from build123d import *

# Parameters (mm, degrees)
BOSS_EXTRUDE1_DEPTH      = 70
BOSS_EXTRUDE1_DEPTH_BACK = 70
SKETCH1_W                = 20
SKETCH1_H                = 10
SKETCH3_W                = 20
SKETCH3_H                = 5
BOSS_EXTRUDE2_DEPTH      = 20
FILLET1_R                = 10
SKETCH4_R                = 2.75
CUT_EXTRUDE1_DEPTH       = 91.863909227
FILLET1_OF_MIRROR1_R     = 10
CHAMFER1_SIZE            = 8.660254038
CHAMFER1_SIZE_2          = 5


# Some blends are built 0.0001 mm under size
with BuildPart() as part:
    # Sketch1 → Boss-Extrude1 (new, two sides: drawn at the far end of the back side and taken through both)
    with BuildSketch(Plane.XY.offset(-BOSS_EXTRUDE1_DEPTH_BACK)):
        Rectangle(SKETCH1_W, SKETCH1_H)
    extrude(amount=BOSS_EXTRUDE1_DEPTH + BOSS_EXTRUDE1_DEPTH_BACK)

    # Sketch3 → Boss-Extrude2 (add)
    with BuildSketch(Plane(origin=(0, 0, -70), x_dir=(-1, 0, 0), z_dir=(0, 0, -1))):
        Rectangle(SKETCH3_W, SKETCH3_H)
    boss_extrude2 = extrude(amount=BOSS_EXTRUDE2_DEPTH)

    # Fillet1
    fillet1_edges = [part.edges().sort_by_distance(p)[0] for p in [
        (-10, 0, -90),
        (10, 0, -90),
    ]]
    fillet(fillet1_edges, radius=FILLET1_R - 0.0001)  # a hair under: the kernel refuses the full size

    # Sketch4 → Cut-Extrude1 (cut, through all)
    with BuildSketch(Plane(origin=(0, 2.5, 0), x_dir=(1, 0, 0), z_dir=(0, 1, 0))):
        with Locations(Location((0, 80, 0), (0, 0, 270))):
            Circle(SKETCH4_R)
    cut_extrude1 = extrude(amount=-CUT_EXTRUDE1_DEPTH, mode=Mode.SUBTRACT)

    # Mirror1: Boss-Extrude2, Cut-Extrude1 across plane
    add(boss_extrude2.mirror(Plane.XY))
    add(cut_extrude1.mirror(Plane.XY), mode=Mode.SUBTRACT)

    # Fillet1 of Mirror1
    fillet1_of_mirror1_edges = [part.edges().sort_by_distance(p)[0] for p in [
        (-10, 0, 90),
        (10, 0, 90),
    ]]
    fillet(fillet1_of_mirror1_edges, radius=FILLET1_OF_MIRROR1_R - 0.0001)  # a hair under: the kernel refuses the full size

    # Chamfer1
    # the kernel refuses this chamfer: 8.660254038, 5 mm, written as the material it takes off along each edge
    with BuildSketch(Plane(origin=(32.404819853, 5, -70), x_dir=(0, 0.019326765612700594, 0.999813220622208), z_dir=(-1, 0, 0))) as chamfer1_piece_1_section:
        Polygon((CHAMFER1_SIZE * 0.999813220604, -CHAMFER1_SIZE * 0.0193267656124), (-CHAMFER1_SIZE_2 * 0.0193267656127, -CHAMFER1_SIZE_2 * 0.999813220622), (0, 0), align=None)
    chamfer1_piece_1 = extrude(amount=64.809639706, mode=Mode.PRIVATE)
    chamfer1_piece_1 = split(chamfer1_piece_1, bisect_by=Plane(origin=(0, 2.5, -66.539331058), z_dir=(0, 1, 0)), keep=Keep.TOP, mode=Mode.PRIVATE)
    add(chamfer1_piece_1, mode=Mode.SUBTRACT)
    with BuildSketch(Plane(origin=(-32.404819853, -5, -70), x_dir=(0, -0.019326765612700594, 0.999813220622208), z_dir=(1, 0, 0))) as chamfer1_piece_2_section:
        Polygon((CHAMFER1_SIZE * 0.999813220604, -CHAMFER1_SIZE * 0.0193267656124), (-CHAMFER1_SIZE_2 * 0.0193267656127, -CHAMFER1_SIZE_2 * 0.999813220622), (0, 0), align=None)
    chamfer1_piece_2 = extrude(amount=64.809639706, mode=Mode.PRIVATE)
    chamfer1_piece_2 = split(chamfer1_piece_2, bisect_by=Plane(origin=(0, -2.5, -66.539331058), z_dir=(0, -1, 0)), keep=Keep.TOP, mode=Mode.PRIVATE)
    add(chamfer1_piece_2, mode=Mode.SUBTRACT)
    with BuildSketch(Plane(origin=(-32.404819853, -5, 70), x_dir=(0, 0.9983227437537926, 0.05789386240267045), z_dir=(1, 0, 0))) as chamfer1_piece_3_section:
        Polygon((CHAMFER1_SIZE_2 * 0.998322743754, -CHAMFER1_SIZE_2 * 0.0578938624027), (-CHAMFER1_SIZE * 0.0578938624016, -CHAMFER1_SIZE * 0.998322743736), (0, 0), align=None)
    chamfer1_piece_3 = extrude(amount=64.809639706, mode=Mode.PRIVATE)
    chamfer1_piece_3 = split(chamfer1_piece_3, bisect_by=Plane(origin=(0, -2.5, 66.539331058), z_dir=(0, -1, 0)), keep=Keep.TOP, mode=Mode.PRIVATE)
    add(chamfer1_piece_3, mode=Mode.SUBTRACT)
    with BuildSketch(Plane(origin=(32.404819853, 5, 70), x_dir=(0, -0.9983227437537926, 0.05789386240267045), z_dir=(-1, 0, 0))) as chamfer1_piece_4_section:
        Polygon((CHAMFER1_SIZE_2 * 0.998322743754, -CHAMFER1_SIZE_2 * 0.0578938624027), (-CHAMFER1_SIZE * 0.0578938624016, -CHAMFER1_SIZE * 0.998322743736), (0, 0), align=None)
    chamfer1_piece_4 = extrude(amount=64.809639706, mode=Mode.PRIVATE)
    chamfer1_piece_4 = split(chamfer1_piece_4, bisect_by=Plane(origin=(0, 2.5, 66.539331058), z_dir=(0, 1, 0)), keep=Keep.TOP, mode=Mode.PRIVATE)
    add(chamfer1_piece_4, mode=Mode.SUBTRACT)


solid = part.part
Check sheet for the modelled part. Datum: model origin and axes. Units: mm. A direction names the side the tool comes from. Coordinates: 2 decimals unless noted, no trailing zeros. Write each loop counter-clockwise with the first axis right and the second up, starting at its lowest first coordinate (ties: lowest second). Pieces come first, ordered by that corner, then holes.
Item 1: Access from +Z, -Z, +X, -X, +Y, -Y to the whole of each face (thin tool, end or side, straight path). Record for faces 1 (the face through (0, 2.5, -75)), 2 (the face through (0, -2.5, -75)), 3 (the face through (0, -2.5, 75)), 4 (the face through (0, 2.5, 75)).
Numbers:
face 1: -Z, +X, -X, +Y
face 2: -Z, +X, -X, -Y
face 3: +Z, +X, -X, -Y
face 4: +Z, +X, -X, +Y
Item 2: Scan lines: probe 1 along X at (y, z) = (0.4, 80); probe 2 along Z at (x, y) = (2.5, 0.25); probe 3 along Y at (x, z) = (7.5, 78.5). Record each from-to range of solid material in increasing order.
Numbers:
probe 1: x = -10 to -2.75, 2.75 to 10
probe 2: z = -89.68 to -81.15, -78.85 to 78.85, 81.15 to 89.68
probe 3: y = -2.5 to 2.5
Item 3: Cross-section at A-A on y = -0.25. Count the separate pieces of the cut face and the enclosed holes in it, then the cut area to 3 significant figures.
Numbers:
separate pieces: 1
enclosed holes: 2
area: 3,470 mm2
Item 4: Cross-section at C-C on x = -4.5. Record the boundary of the cut face in (y, z).
Numbers:
outline: (-5, -61.34) - (-2.5, -65.67) - (-2.5, -88.93) - (2.5, -88.93) - (2.5, -65.67) - (5, -61.34) - (5, 61.34) - (2.5, 65.67) - (2.5, 88.93) - (-2.5, 88.93) - (-2.5, 65.67) - (-5, 61.34) - close
Item 5: Depth check by flat-ended pin: pin 1 Ø4 at (x, y) = (2.5, 3) entering from -Z; pin 2 Ø6 at (x, z) = (1, -80) entering from -Y; pin 3 Ø6.5 at (x, z) = (0, 80) entering from +Y. Enter the tip coordinate at first touch or a pass-through.
Numbers:
pin 1: stops at z = -89.98
pin 2: stops at y = -2.5
pin 3: stops at y = 2.5
Item 6: Mould release check, pull along Z, two halves, no side actions. Record for faces 5 (the face through (0.121, 0.035, 82.747)), 6 (the face through (7.15, 0.04, -86.99)), 7 (the face through (0, -5, -1)): released by +Z, released by -Z, zero draft, split by the parting line, or undercut.
Numbers:
face 5: undercut
face 6: released by -Z
face 7: zero draft
Item 7: Cross-section at B-B on x = 6.75. Record the boundary of the cut face in (y, z).
Numbers:
outline: (-5, -61.34) - (-2.5, -65.67) - (-2.5, -87.38) - (2.5, -87.38) - (2.5, -65.67) - (5, -61.34) - (5, 61.34) - (2.5, 65.67) - (2.5, 87.38) - (-2.5, 87.38) - (-2.5, 65.67) - (-5, 61.34) - close
